```python
from build123d import *

# Parameters (mm, degrees)
F0_R           = 86.0425
F1_DEPTH       = 11.938
F2_R           = 61.722
F3_DEPTH       = 13.462
F5_DEPTH       = 25.401
F7_D           = 5.99948
F7_CBORE_D     = 11.00074
F7_CBORE_DEPTH = 6.35
F9_D           = 10.71626


with BuildPart() as f1:
    # F0 (on Front) → F1 (new body)
    with BuildSketch(Plane.XZ):
        Circle(F0_R)
    extrude(amount=F1_DEPTH)

    # F2 (on face) → F3 (join)
    with BuildSketch(Plane(origin=(0, 0, 0), x_dir=(-1, 0, 0), z_dir=(0, 1, 0))):
        Circle(F2_R)
    extrude(amount=F3_DEPTH)

    # F4 (on face) → F5 (cut, through all)
    with BuildSketch(Plane.XZ.offset(11.938)):
        with BuildLine():
            Line((-85.9716026302, -3.4921837637), (-39.9614814611, 76.1996837637))
            ThreePointArc((-39.9614814611, 76.1996837637), (-74.5149908051, 43.02125), (-85.9716026302, -3.4921837637))
        make_face()
        with BuildLine():
            ThreePointArc((86.0425, 0), (73.6264136532, 44.5248584368), (39.9614814611, 76.1996837637))
            Line((39.9614814611, 76.1996837637), (85.9716026302, -3.4921837637))
            ThreePointArc((85.9716026302, -3.4921837637), (86.0247738316, -1.7464516796), (86.0425, 0))
        make_face()
        with BuildLine():
            ThreePointArc((-46.0101211692, -72.7075), (0, -86.0425), (46.0101211692, -72.7075))
            Line((46.0101211692, -72.7075), (-46.0101211692, -72.7075))
        make_face()
    extrude(amount=-F5_DEPTH, mode=Mode.SUBTRACT)

    # F7 (through all)
    with Locations(Plane.XZ.offset(11.938)):
        with Locations((20.193, 75.2348), (-20.193, 75.2348), (-75.1715490214, -20.2099480486), (-54.9785490214, -55.1852500059), (55.1683019572, -55.0756960973), (75.3613019572, -20.10039414)):
            CounterBoreHole(F7_D / 2, F7_CBORE_D / 2, F7_CBORE_DEPTH)

    # F9 (through all)
    with Locations(Plane.XZ.offset(11.938)):
        with Locations((0, 0)):
            Hole(F9_D / 2)


solid = f1.part
```
Build history of the part. All positions in model axes, mm. A direction names the side the tool comes from. Give positions to 0.01 mm unless a question says otherwise; leave off trailing zeros. Loops run counter-clockwise (first coordinate to the right, second up) from the corner with the lowest first, then second, coordinate; pieces in that order, holes last. Notation, with made-up numbers: (82, 55.5) -> (88, 55.5) arc R32 cw to (88, 82.5) -> close; hole circle Ø7 at (86.25, 52.5). An arc over 180 degrees is marked (long way). One line per question, with ' | ' between items. Start each with the question number.
1) Two-plate mould, pull along X, no slides. Class faces 1 (the flat face through (6, 0, -64)), 2 (the cylindrical face through (19.001, -8.807, 69.865)), 3 (the cylindrical face through (-74.8, -5.89, -42.52)): released by +X, released by -X, zero draft, split by the parting line, or undercut.
2) Cut at B-B (z = 0). Give the cut face in (x, y), plus the area to 3 significant figures.
3) Cut at A-A (x = 0). Give the cut face in (y, z).
4) 3-axis set-ups, long thin cutter, end or side, ignore diameter. For faces 4 (the flat face through (-17.8, -5.588, 72.9)), 5 (the cylindrical face through (0.58, -5.89, 86.04)), 6 (the cylindrical face through (8, 6.6, 61.2)): which of +Z, -Z, +X, -X, +Y, -Y reach the whole face in a straight line?
5) Pin check, flat tips, straight feed: pin 1 (3.5 mm diameter, centred on x = 75.36, z = -20.1, fed in from -Y); pin 2 (6.5 mm diameter, centred on x = -20.19, z = 75.23, fed in from -Y); pin 3 (1 mm diameter, centred on y = -7.5, z = -11.5, fed in from -X); pin 4 (3 mm diameter, centred on x = -8.5, y = -6.5, fed in from +Z). Stop position of each tip, or through.
6) Probe L1, parallel to Y at x = -59, z = -62.5; L2, parallel to Z at x = -73, y = -10.5; L3, parallel to Z at x = -74, y = -4. List the from-to ranges inside material, lowest first.
7) Cut at C-C (y = 3.5). Give the cut face in (x, z), plus the area to 3 significant figures.
8) Cut at D-D (z = 41.5). Give the cut face in (x, y).
Return value:
1) face 1: zero draft | face 2: undercut | face 3: released by -X
2) outline: (-83.96, -11.94) -> (-5.36, -11.94) -> (-5.36, 13.46) -> (-61.72, 13.46) -> (-61.72, 0) -> (-83.96, 0) -> close; (5.36, -11.94) -> (83.96, -11.94) -> (83.96, 0) -> (61.72, 0) -> (61.72, 13.46) -> (5.36, 13.46) -> close | area: 3,390 mm^2
3) outline: (-11.94, -72.71) -> (0, -72.71) -> (0, -61.72) -> (13.46, -61.72) -> (13.46, -5.36) -> (-11.94, -5.36) -> close; (-11.94, 5.36) -> (13.46, 5.36) -> (13.46, 61.72) -> (0, 61.72) -> (0, 86.04) -> (-11.94, 86.04) -> close
4) face 4: -Y | face 5: +Z, +Y, -Y | face 6: +Y
5) pin 1: through | pin 2: y = -5.59 | pin 3: x = -85.34 | pin 4: z = 85.76
6) L1: -11.94 to 0 | L2: -45.54 to -25.26, -15.16 to 18.98 | L3: -43.9 to -22.97, -17.45 to 17.24
7) outline: circle Ø123.44 at (0, 0); hole circle Ø10.72 at (0, 0) | area: 11,900 mm^2
8) outline: (-60, -11.94) -> (60, -11.94) -> (60, 0) -> (45.69, 0) -> (45.69, 13.46) -> (-45.69, 13.46) -> (-45.69, 0) -> (-60, 0) -> close
